Verification items for the finished model (mm, model axes). Face numbers are marked on the shaded views. A direction names the side the tool comes from. Coordinates: 2 decimals unless noted, no trailing zeros. Loops run counter-clockwise (first coordinate to the right, second up) from the corner with the lowest first, then second, coordinate; pieces in that order, holes last.
Q1. Sectioned sample at B-B (y = 0). Enter the section's corners in (x, z) (3 decimals), then the cut area to 3 significant figures.
Q2. Sectioned sample at D-D (x = -2.5). Enter the section's corners in (y, z), then the cut area to 3 significant figures.
Q3. Sectioned sample at C-C (z = 26). Enter the section's corners in (x, y).
Q4. Sectioned sample at A-A (x = 0). Count the separate pieces of the cut face and the enclosed holes in it, then the cut area to 3 significant figures.
Q5. Material ranges on probe 1 along Z at (x, y) = (0.25, 2.25); probe 2 along Y at (x, z) = (0.75, 34); probe 3 along X at (y, z) = (1.25, 21), recorded low to high.
Q6. Go/stop test with flat-tipped pins: P1, Ø1.7, axis at x = 0, z = 15.82, coming from the -Y side; P2, Ø3, axis at x = 2, z = 24, coming from the +Y side; P3, Ø2, axis at x = 0, z = 3.32, coming from the +Y side. Record where each tip stops, or that it passes through.
Q7. Access from +Z, -Z, +X, -X, +Y, -Y to the whole of each face (thin tool, end or side, straight path). Record for the marked faces 1, 2 and 3.
```python
from build123d import *

# Parameters (mm, degrees)
F0_R     = 2
F1_DEPTH = 32
F2_R     = 3.44
F2_R_2   = 2
F3_DEPTH = 0.5
F4_R     = 1.665
F5_DEPTH = 5
F7_R     = 0.75
F8_DEPTH = 10


with BuildPart() as f1:
    # F0 (on Top) → F1 (new body)
    with BuildSketch(Plane.XY):
        Circle(F0_R)
    extrude(amount=F1_DEPTH)

    # F2 (on face) → F3 (join)
    with BuildSketch(Plane.XY.offset(32)):
        Circle(F2_R)
        Circle(F2_R_2, mode=Mode.SUBTRACT)
        Circle(F2_R_2)
    extrude(amount=F3_DEPTH)

    # F4 (on face) → F5 (join)
    with BuildSketch(Plane.XY.offset(32.5)):
        Circle(F4_R)
    extrude(amount=F5_DEPTH)

    # F7 (on offset) → F8 (cut)
    with BuildSketch(Plane.XZ.offset(4)):
        with Locations((0, 3.3206201717)):
            Circle(F7_R)
        with Locations((0, 5.8206201717)):
            Circle(F7_R)
        with Locations((0, 8.3206201717)):
            Circle(F7_R)
        with Locations((0, 10.8206201717)):
            Circle(F7_R)
        with Locations((-0.0019225008, 35.2506788733)):
            Circle(F7_R)
        with Locations((0, 13.3206201717)):
            Circle(F7_R)
        with Locations((0, 15.8206201717)):
            Circle(F7_R)
    extrude(amount=-F8_DEPTH, mode=Mode.SUBTRACT)


solid = f1.part
```
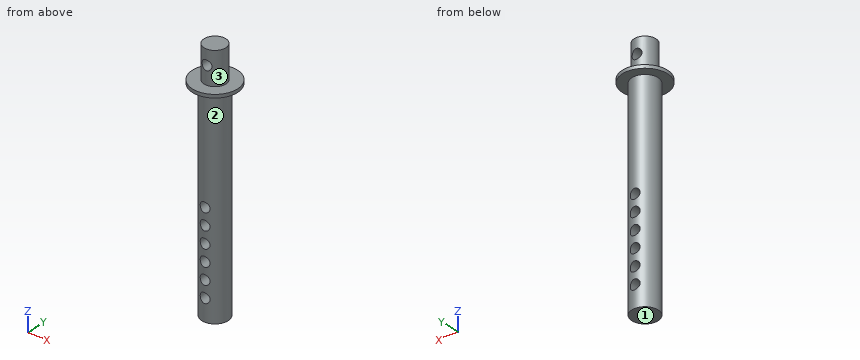
Geometry check:
1. outline: (-3.44, 32) - (-2, 32) - (-2, 0) - (2, 0) - (2, 32) - (3.44, 32) - (3.44, 32.5) - (1.665, 32.5) - (1.665, 37.5) - (-1.665, 37.5) - (-1.665, 32.5) - (-3.44, 32.5) - close; hole circle Ø1.5 at (-0.002, 35.251); hole circle Ø1.5 at (0, 3.321); hole circle Ø1.5 at (0, 5.821); hole circle Ø1.5 at (0, 8.321); hole circle Ø1.5 at (0, 10.821); hole circle Ø1.5 at (0, 13.321); hole circle Ø1.5 at (0, 15.821)
1. area: 136 mm2
2. outline: (-2.36, 32) - (2.36, 32) - (2.36, 32.5) - (-2.36, 32.5) - close
2. area: 2.36 mm2
3. outline: circle Ø4 at (0, 0)
4. separate pieces: 8
4. enclosed holes: 0
4. area: 107 mm2
5. probe 1: z = 32 to 32.5
5. probe 2: y = -1.49 to 1.49
5. probe 3: x = -1.56 to 1.56
6. P1: stops at y = -2
6. P2: stops at y = 1.94
6. P3: stops at y = 2
7. face 1: -Z, +X, -X, +Y, -Y
7. face 2: -Z
7. face 3: +Z
